The listing builds one solid part. Answer for the finished solid, in the listing's coordinates (mm). A direction names the side the tool comes from. Give positions to 0.01 mm unless a question says otherwise; leave off trailing zeros. Write each loop counter-clockwise with the first axis right and the second up, starting at its lowest first coordinate (ties: lowest second). Pieces come first, ordered by that corner, then holes. Notation, with made-up numbers: (-39.5, 17) - (-11.5, 17) arc R14 cw to (-11.5, 29) - close; hole circle Ø8 at (-20.75, 64.25). An arc over 180 degrees is marked (long way). Write each question's results on one line, items separated by ' | '. Start each with the question number.
Q1. Flat-ended cylindrical pins translate along their axes: pin 1 Ø6 at (x, z) = (6.5, 5.5) entering from +Y; pin 2 Ø2 at (y, z) = (-36.5, 22.5) entering from -X; pin 3 Ø3.5 at (y, z) = (-42.33, 8) entering from +X; pin 4 Ø7 at (y, z) = (-8.5, 14.5) entering from +X. Find the tip coordinate at first contact, or state that the pin passes through.
Q2. For a pull along Y with two mould halves and no side action, classify faces 1 (the face through (-21, 0, 15)), 2 (the face through (36, -27.33, 15)), 3 (the face through (52.776, -44.177, 21.234)) as pulls with the +Y half, pulls with the -Y half, needs draft (parallel to the pull), parting line crosses it, or undercut.
Q3. Section A-A (z = 8) is taken. Determine the outline of the cut face in (x, y), plus the area to 3 significant figures.
Q4. For faces 4 (the face through (-23, -12, 15)), 5 (the face through (-19.692, -30.863, 14.79)), 6 (the face through (37, -23, 15)), 7 (the face through (18.132, -32.132, 14.79)), 8 (the face through (0, -31, 15)), determine the directions among +Z, -Z, +X, -X, +Y, -Y from which every point of the face is accessible in a straight line to the end or side of a thin tool.
Q5. Find the intervals of material crossed by probe 1 along X at (y, z) = (-3.5, 14); probe 2 along Y at (x, z) = (36, 1.75); probe 3 along Y at (x, z) = (-12, 26.75), in increasing order.
Q6. Section C-C (y = -6) is taken. Determine the outline of the cut face in (x, z), plus the area to 3 significant figures.
Q7. Section D-D (z = 27) is taken. Determine the outline of the cut face in (x, y).
Q8. Section B-B (y = -29.5) is taken. Determine the outline of the cut face in (x, z).
```python
from build123d import *

# Parameters (mm, degrees)
BOSS_EXTRUDE1_DEPTH = 30
BOSS_EXTRUDE2_DEPTH = 30
SKETCH3_W           = 3
SKETCH3_H           = 30
BOSS_EXTRUDE3_DEPTH = 30
FILLET1_R           = 1
FILLET2_R           = 2
SKETCH4_R           = 2
CUT_EXTRUDE1_DEPTH  = 30
FILLET3_R           = 2
SKETCH6_W           = 80.718838425
SKETCH6_H           = 35.980410733
CUT_EXTRUDE2_DEPTH  = 84.819501439


with BuildPart() as part:
    # Sketch1 → Boss-Extrude1 (new body)
    with BuildSketch(Plane.XY):
        with BuildLine():
            Line((-12, 34), (12, 34))
            ThreePointArc((12, 34), (19.778174593, 30.778174593), (23, 23))
            Line((23, 23), (23, -23))
            ThreePointArc((23, -23), (19.778174593, -30.778174593), (12, -34))
            Line((12, -34), (-12, -34))
            ThreePointArc((-12, -34), (-19.778174593, -30.778174593), (-23, -23))
            Line((-23, -23), (-23, 23))
            ThreePointArc((-23, 23), (-19.778174593, 30.778174593), (-12, 34))
        make_face()
        with BuildLine():
            Line((-12, 31), (12, 31))
            ThreePointArc((12, 31), (17.656854249, 28.656854249), (20, 23))
            Line((20, 23), (20, -23))
            ThreePointArc((20, -23), (17.656854249, -28.656854249), (12, -31))
            Line((12, -31), (-12, -31))
            ThreePointArc((-12, -31), (-17.656854249, -28.656854249), (-20, -23))
            Line((-20, -23), (-20, 23))
            ThreePointArc((-20, 23), (-17.656854249, 28.656854249), (-12, 31))
        make_face(mode=Mode.SUBTRACT)
    extrude(amount=BOSS_EXTRUDE1_DEPTH)

    # Sketch2 → Boss-Extrude2 (add)
    with BuildSketch(Plane.XY):
        with BuildLine():
            Line((23, -23), (53.282521301, -23))
            Line((53.282521301, -23), (53.282521301, -27.329588742))
            Line((53.282521301, -27.329588742), (22.112104693, -27.329588742))
            ThreePointArc((22.112104693, -27.329588742), (22.775740151, -25.209847096), (23, -23))
        make_face()
    extrude(amount=BOSS_EXTRUDE2_DEPTH)

    # Sketch3 → Boss-Extrude3 (add)
    with BuildSketch(Plane.XZ.offset(27.329588742)):
        with Locations((51.782521301, 15)):
            Rectangle(SKETCH3_W, SKETCH3_H)
    extrude(amount=BOSS_EXTRUDE3_DEPTH)

    # Fillet1
    fillet1_edges = [part.edges().sort_by_distance(p)[0] for p in [
        (50.282521301, -27.329588742, 15),
    ]]
    fillet(fillet1_edges, radius=FILLET1_R)

    # Fillet2
    fillet2_edges = [part.edges().sort_by_distance(p)[0] for p in [
        (53.282521301, -23, 15),
    ]]
    fillet(fillet2_edges, radius=FILLET2_R)

    # Sketch4 → Cut-Extrude1 (cut)
    with BuildSketch(Plane.ZY.offset(-50.282521301)):
        with Locations(Location((22, -42.329588742, 0), (0, 0, 270))):
            Circle(SKETCH4_R)
        with Locations(Location((8, -42.329588742, 0), (0, 0, 270))):
            Circle(SKETCH4_R)
    extrude(amount=-CUT_EXTRUDE1_DEPTH, mode=Mode.SUBTRACT)

    # Fillet3
    fillet3_edges = [part.edges().sort_by_distance(p)[0] for p in [
        (50.282521301, -40.329588742, 22),
        (50.282521301, -40.329588742, 8),
    ]]
    fillet(fillet3_edges, radius=FILLET3_R)

    # Sketch6 → Cut-Extrude2 (cut, through all)
    with BuildSketch(Plane(origin=(0, 0, 0), x_dir=(-1, 0, 0), z_dir=(0, 0, -1))):
        with Locations((3.744263304, 17.990205366)):
            Rectangle(SKETCH6_W, SKETCH6_H)
    extrude(amount=-CUT_EXTRUDE2_DEPTH, mode=Mode.SUBTRACT)


solid = part.part
```
Answers below:
1) pin 1: stops at y = -31 | pin 2: stops at x = 50.28 | pin 3: passes through | pin 4: stops at x = 23
2) face 1: pulls with the +Y half | face 2: pulls with the -Y half | face 3: undercut
3) outline: (-23, -23) arc R11 ccw to (-12, -34) - (12, -34) arc R11 ccw to (22.11, -27.33) - (49.28, -27.33) arc R1 cw to (50.28, -28.33) - (50.28, -38.33) arc R2 ccw to (52.28, -40.33) - (53.28, -40.33) - (53.28, -25) arc R2 ccw to (51.28, -23) - (23, -23) - (23, 0) - (20, 0) - (20, -23) arc R8 cw to (12, -31) - (-12, -31) arc R8 cw to (-20, -23) - (-20, 0) - (-23, 0) - close; (50.28, -57.33) - (53.28, -57.33) - (53.28, -44.33) - (52.28, -44.33) arc R2 ccw to (50.28, -46.33) - close | area: 508 mm2
4) face 4: +Z, -Z, -X, +Y, -Y | face 5: +Z, -Z, -X, -Y | face 6: +Z, -Z, +X, +Y | face 7: +Z, -Z, -Y | face 8: +Z, -Z, +Y
5) probe 1: x = -23 to -20, 20 to 23 | probe 2: y = -27.33 to -23 | probe 3: y = -34 to -31
6) outline: (-23, 0) - (-20, 0) - (-20, 30) - (-23, 30) - close; (20, 0) - (23, 0) - (23, 30) - (20, 30) - close | area: 180 mm2
7) outline: (-23, -23) arc R11 ccw to (-12, -34) - (12, -34) arc R11 ccw to (22.11, -27.33) - (49.28, -27.33) arc R1 cw to (50.28, -28.33) - (50.28, -57.33) - (53.28, -57.33) - (53.28, -25) arc R2 ccw to (51.28, -23) - (23, -23) - (23, 0) - (20, 0) - (20, -23) arc R8 cw to (12, -31) - (-12, -31) arc R8 cw to (-20, -23) - (-20, 0) - (-23, 0) - close
8) outline: (-20.87, 0) - (-16.66, 0) - (-16.66, 30) - (-20.87, 30) - close; (16.66, 0) - (20.87, 0) - (20.87, 30) - (16.66, 30) - close; (50.28, 0) - (53.28, 0) - (53.28, 30) - (50.28, 30) - close
